```python
from build123d import *

# Parameters (mm, degrees)
SKETCH_1_R          = 17
EXTRUDE_1_DEPTH     = 33
SKETCH_2_R          = 18.5
EXTRUDE_2_DEPTH     = 22
EXTRUDE_3_DEPTH     = 1.8
SKETCH_4_W          = 42
SKETCH_4_H          = 1.9
EXTRUDE_4_DEPTH     = 39
SKETCH_5_R          = 6
EXTRUDE_5_DEPTH     = 4
SKETCH_6_R          = 3
EXTRUDE_6_DEPTH     = 15
CUT_EXTRUDE_1_REACH = 67.558
SKETCH_7_R          = 1.7


with BuildPart() as part:
    # 草图1 → 凸台-拉伸1 (new body)
    with BuildSketch(Plane(origin=(0, 0, 0), x_dir=(1, 0, 0), z_dir=(0, 1, 0))):
        with Locations(Location((0, 0, 0), (0, 0, 270))):
            Circle(SKETCH_1_R)
    extrude(amount=EXTRUDE_1_DEPTH)

    # 草图2 → 凸台-拉伸2 (add)
    with BuildSketch(Plane.XZ):
        with Locations(Location((0, 0, 0), (0, 0, 270))):
            Circle(SKETCH_2_R)
    extrude(amount=EXTRUDE_2_DEPTH)

    # 草图3 → 凸台-拉伸3 (add)
    with BuildSketch(Plane.XZ.offset(22)):
        with BuildLine():
            Line((-21, 0), (-21, -24))
            Line((-21, -24), (21, -24))
            Line((21, -24), (21, 0))
            ThreePointArc((21, 0), (0, 21), (-21, 0))
        make_face()
    extrude(amount=EXTRUDE_3_DEPTH)

    # 草图4 → 凸台-拉伸4 (add)
    with BuildSketch(Plane(origin=(0, -22, 0), x_dir=(1, 0, 0), z_dir=(0, 1, 0))):
        with Locations((0, 23.05)):
            Rectangle(SKETCH_4_W, SKETCH_4_H)
    extrude(amount=EXTRUDE_4_DEPTH)

    # 草图5 → 凸台-拉伸5 (add)
    with BuildSketch(Plane.XZ.offset(23.8)):
        with Locations(Location((0, -1.8, 0), (0, 0, 270))):
            Circle(SKETCH_5_R)
    extrude(amount=EXTRUDE_5_DEPTH)

    # 草图6 → 凸台-拉伸6 (add)
    with BuildSketch(Plane.XZ.offset(27.8)):
        with Locations(Location((0, -1.8, 0), (0, 0, 270))):
            Circle(SKETCH_6_R)
    extrude(amount=EXTRUDE_6_DEPTH)

    # 草图7 → 切除-拉伸1 (cut, up to next)
    with BuildSketch(Plane(origin=(0, 0, -24), x_dir=(-1, 0, 0), z_dir=(0, 0, -1)), mode=Mode.PRIVATE) as cut_extrude_1_sk1:
        with Locations((-15, 8.35)):
            Circle(SKETCH_7_R)
    cut_extrude_1_tool1 = extrude(cut_extrude_1_sk1.sketch, amount=-CUT_EXTRUDE_1_REACH, mode=Mode.PRIVATE) & part.part
    # 草图7 → 切除-拉伸1 (cut, up to next)
    with BuildSketch(Plane(origin=(0, 0, -24), x_dir=(-1, 0, 0), z_dir=(0, 0, -1)), mode=Mode.PRIVATE) as cut_extrude_1_sk2:
        with Locations((-15, -15.65)):
            Circle(SKETCH_7_R)
    cut_extrude_1_tool2 = extrude(cut_extrude_1_sk2.sketch, amount=-CUT_EXTRUDE_1_REACH, mode=Mode.PRIVATE) & part.part
    # 草图7 → 切除-拉伸1 (cut, up to next)
    with BuildSketch(Plane(origin=(0, 0, -24), x_dir=(-1, 0, 0), z_dir=(0, 0, -1)), mode=Mode.PRIVATE) as cut_extrude_1_sk3:
        with Locations((15, 8.35)):
            Circle(SKETCH_7_R)
    cut_extrude_1_tool3 = extrude(cut_extrude_1_sk3.sketch, amount=-CUT_EXTRUDE_1_REACH, mode=Mode.PRIVATE) & part.part
    # 草图7 → 切除-拉伸1 (cut, up to next)
    with BuildSketch(Plane(origin=(0, 0, -24), x_dir=(-1, 0, 0), z_dir=(0, 0, -1)), mode=Mode.PRIVATE) as cut_extrude_1_sk4:
        with Locations((15, -15.65)):
            Circle(SKETCH_7_R)
    cut_extrude_1_tool4 = extrude(cut_extrude_1_sk4.sketch, amount=-CUT_EXTRUDE_1_REACH, mode=Mode.PRIVATE) & part.part
    add(cut_extrude_1_tool1.solids().sort_by_distance((15, 8.35, -24))[0], mode=Mode.SUBTRACT)
    add(cut_extrude_1_tool2.solids().sort_by_distance((15, -15.65, -24))[0], mode=Mode.SUBTRACT)
    add(cut_extrude_1_tool3.solids().sort_by_distance((-15, 8.35, -24))[0], mode=Mode.SUBTRACT)
    add(cut_extrude_1_tool4.solids().sort_by_distance((-15, -15.65, -24))[0], mode=Mode.SUBTRACT)


solid = part.part
```
The listing builds one solid part. Answer for the finished solid, in the listing's coordinates (mm). A direction names the side the tool comes from. Round coordinates to 2 decimals unless told otherwise and drop trailing zeros. Write each loop counter-clockwise with the first axis right and the second up, starting at its lowest first coordinate (ties: lowest second). Pieces come first, ordered by that corner, then holes. Notation, with made-up numbers: (-29, -7.75) -> (25, -7.75) arc R6 cw to (25, 1.25) -> close; hole circle Ø11 at (55.5, 32). An arc over 180 degrees is marked (long way). Answer as a JSON object with one key per item and string values. Group by question number.
Q1. Determine the mould class of faces 5 (the face through (-15.78, -17.16, -23.06)), 6 (the face through (-16.57, 7.7, -23.06)), 7 (the face through (-2.3, -25.77, -7.34)), 8 (the face through (4.4, -23.8, -6.2)) for opening direction X: pulls with the +X half, pulls with the -X half, needs draft (parallel to the pull), parting line crosses it, or undercut.
Q2. Straight lines are drawn through the part: line 1 along Y through (x, z) = (15, -22.8); line 2 along Y through (x, z) = (-15.5, 9); line 3 along X through (y, z) = (-15, -23). For each, find the intervals that lie inside material, in ascending order.
Q3. Which of the six approach directions +Z, -Z, +X, -X, +Y, -Y give full straight-line access (tool end or side, diameter ignored) to faces 1 (the face through (0, -3, -22.1)), 2 (the face through (0.1, -35.2, 1.2)), 3 (the face through (16.855, 16.269, -2.213)), 4 (the face through (0, 17, -23))?
Q4. Section D-D (y = -18.5) is taken. Write down the section's boundary in (x, z), plus the area to 3 significant figures.
Q5. Section B-B (x = 0) is taken. Write down the section's boundary in (y, z), plus the area to 3 significant figures.
Q6. Section C-C (x = 15.5) is taken. Write down the section's boundary in (y, z), plus the area to 3 significant figures.
Q7. Each of these flat-tipped pins is pushed along its axis until it touches: pin 1 Ø4 at (y, z) = (-13.5, 8.5) entering from +X; pin 2 Ø4 at (x, y) = (15, 8.35) entering from +Z; pin 3 Ø10 at (y, z) = (-27, 5.5) entering from -X. Where does it stop, or does it pass through?
Q8. Section A-A (y = 8.35) is taken. Write down the section's boundary in (x, z), plus the area to 3 significant figures.
Check values:
{
 "1": {"face 5": "undercut", "face 6": "undercut", "face 7": "parting line crosses it", "face 8": "needs draft"},
 "2": {"line 1": "-23.8 to -17.35, -13.95 to 6.65, 10.05 to 17", "line 2": "-23.8 to 0", "line 3": "-21 to -16.57, -13.43 to 13.43, 16.57 to 21"},
 "3": {"face 1": "+X, -X, +Y", "face 2": "-Y", "face 3": "+Y", "face 4": "-Z, +X, -X, +Y"},
 "4": {"outline": "(-21, -24) -> (21, -24) -> (21, -22.1) -> (-21, -22.1) -> close; circle Ø37 at (0, 0)", "area": "1,160 mm^2"},
 "5": {"outline": "(-42.8, -4.8) -> (-27.8, -4.8) -> (-27.8, -7.8) -> (-23.8, -7.8) -> (-23.8, -24) -> (17, -24) -> (17, -22.1) -> (-22, -22.1) -> (-22, -18.5) -> (0, -18.5) -> (0, -17) -> (33, -17) -> (33, 17) -> (0, 17) -> (0, 18.5) -> (-22, 18.5) -> (-22, 21) -> (-23.8, 21) -> (-23.8, 4.2) -> (-27.8, 4.2) -> (-27.8, 1.2) -> (-42.8, 1.2) -> close", "area": "2,230 mm^2"},
 "6": {"outline": "(-23.8, -24) -> (-17.27, -24) -> (-17.27, -22.1) -> (-22, -22.1) -> (-22, -10.1) -> (0, -10.1) -> (0, -6.98) -> (33, -6.98) -> (33, 6.98) -> (0, 6.98) -> (0, 10.1) -> (-22, 10.1) -> (-22, 14.17) -> (-23.8, 14.17) -> close; (-14.03, -24) -> (6.73, -24) -> (6.73, -22.1) -> (-14.03, -22.1) -> close; (9.97, -24) -> (17, -24) -> (17, -22.1) -> (9.97, -22.1) -> close", "area": "1,040 mm^2"},
 "7": {"pin 1": "x = 17.32", "pin 2": "z = 10.95", "pin 3": "x = -20.93"},
 "8": {"outline": "(-21, -24) -> (-16.7, -24) -> (-16.7, -22.1) -> (-21, -22.1) -> close; circle Ø34 at (0, 0); (-13.3, -24) -> (13.3, -24) -> (13.3, -22.1) -> (-13.3, -22.1) -> close; (16.7, -24) -> (21, -24) -> (21, -22.1) -> (16.7, -22.1) -> close", "area": "975 mm^2"}
}
